```python
from build123d import *

# Parameters (mm, degrees)
SKETCH8_W           = 75
SKETCH8_H           = 10
BOSS_EXTRUDE5_DEPTH = 10
SKETCH9_R           = 5
BOSS_EXTRUDE7_DEPTH = 25
CUT_EXTRUDE1_DEPTH  = 84.366660003
CHAMFER1_SIZE       = 1
FILLET1_R           = 1


with BuildPart() as part:
    # Sketch8 → Boss-Extrude5 (new body)
    with BuildSketch(Plane(origin=(0, 0, 0), x_dir=(1, 0, 0), z_dir=(0, 1, 0))):
        with Locations((-37.5, -5)):
            Rectangle(SKETCH8_W, SKETCH8_H)
    extrude(amount=BOSS_EXTRUDE5_DEPTH)

    # Sketch9 → Boss-Extrude7 (add)
    with BuildSketch(Plane(origin=(0, 10, 0), x_dir=(1, 0, 0), z_dir=(0, 1, 0))):
        with Locations(Location((-70, -5, 0), (0, 0, 270))):
            Circle(SKETCH9_R)
    extrude(amount=BOSS_EXTRUDE7_DEPTH)

    # Sketch13 → Cut-Extrude1 (cut, through all)
    with BuildSketch(Plane.XY.offset(10)):
        with BuildLine():
            Line((-3.73, 6.977270846), (-6.27, 6.977270846))
            ThreePointArc((-6.27, 6.977270846), (-6.126499001, 2.937598487), (-2.65, 5))
            ThreePointArc((-2.65, 5), (-2.937598487, 6.126499001), (-3.73, 6.977270846))
        make_face()
    extrude(amount=-CUT_EXTRUDE1_DEPTH, mode=Mode.SUBTRACT)

    # Chamfer1
    # the kernel refuses this chamfer: 1 mm, written as the material it takes off along each edge
    with BuildSketch(Plane(origin=(-74.333333333, 9.333333333, 0.666666667), x_dir=(-0.7071067811865476, 0, 0.7071067811865475), z_dir=(-0.5773502691896257, 0.5773502691896256, -0.5773502691896258)), Plane(origin=(-74.333333333, 9.333333333, 9.333333333), x_dir=(0, 0.7071067811865475, -0.7071067811865475), z_dir=(-0.5773502691896258, 0.5773502691896258, 0.5773502691896258)), Plane(origin=(-0.666666667, 9.333333333, 9.333333333), x_dir=(0.7071067811865479, 0, -0.7071067811865471), z_dir=(0.5773502691896254, 0.577350269189626, 0.577350269189626)), Plane(origin=(-74.333333333, 0.666666667, 0.666666667), x_dir=(0, -0.7071067811865476, 0.7071067811865476), z_dir=(-0.5773502691896256, -0.5773502691896258, -0.5773502691896258)), Plane(origin=(-0.666666667, 0.666666667, 0.666666667), x_dir=(0.7071067811865476, 0, 0.7071067811865475), z_dir=(0.5773502691896257, -0.5773502691896257, -0.5773502691896258))) as chamfer1_piece_1:
        Polygon((-0.707106781, -0.40824829), (0.707106781, -0.40824829), (0, 0.816496581), align=None)
    extrude(amount=1.270170592, mode=Mode.SUBTRACT)
    with BuildSketch(Plane(origin=(-0.666666667, 9.333333333, 0.666666667), x_dir=(0.7071067811865476, 0, 0.7071067811865475), z_dir=(0.5773502691896257, 0.5773502691896257, -0.5773502691896258)), Plane(origin=(-74.333333333, 0.666666667, 9.333333333), x_dir=(0, -0.7071067811865475, -0.7071067811865476), z_dir=(-0.5773502691896256, -0.5773502691896258, 0.5773502691896257)), Plane(origin=(-0.666666667, 0.666666667, 9.333333333), x_dir=(0.7071067811865479, 0, -0.7071067811865471), z_dir=(0.5773502691896253, -0.577350269189626, 0.5773502691896258))) as chamfer1_piece_2:
        Polygon((-0.707106781, 0.40824829), (0.707106781, 0.40824829), (0, -0.816496581), align=None)
    extrude(amount=1.270170592, mode=Mode.SUBTRACT)
    with BuildSketch(Plane(origin=(-75, 10, -2.571682988), x_dir=(-0.0274958766105822, -0.999621916911297, 0), z_dir=(0, 0, 1))) as chamfer1_piece_3_section:
        Polygon((CHAMFER1_SIZE * 0.999621916911, CHAMFER1_SIZE * 0.0274958766106), (-CHAMFER1_SIZE * 0.0274958766106, CHAMFER1_SIZE * 0.999621916911), (0, 0), align=None)
    chamfer1_piece_3 = extrude(amount=7.571682988, mode=Mode.PRIVATE)
    chamfer1_piece_3 = chamfer1_piece_3 - Plane(origin=(-70, 9.64391603, 5), x_dir=(0, 0, 1), z_dir=(0, -1, 0)) * Cylinder(5, 20, mode=Mode.PRIVATE)
    add(chamfer1_piece_3, mode=Mode.SUBTRACT)
    with BuildSketch(Plane(origin=(-77.571682988, 10, 10), x_dir=(0, -0.9996219169112968, 0.027495876610585647), z_dir=(1, 0, 0))) as chamfer1_piece_4_section:
        Polygon((CHAMFER1_SIZE * 0.999621916911, CHAMFER1_SIZE * 0.0274958766106), (-CHAMFER1_SIZE * 0.0274958766106, CHAMFER1_SIZE * 0.999621916911), (0, 0), align=None)
    chamfer1_piece_4 = extrude(amount=7.571682988, mode=Mode.PRIVATE)
    chamfer1_piece_4 = chamfer1_piece_4 - Plane(origin=(-70, 9.64391603, 5), x_dir=(0, 0, 1), z_dir=(0, -1, 0)) * Cylinder(5, 20, mode=Mode.PRIVATE)
    add(chamfer1_piece_4, mode=Mode.SUBTRACT)
    with BuildSketch(Plane(origin=(-69.999999992, 10, 0), x_dir=(0, -0.9996219169112968, -0.0274958766105864), z_dir=(-1, 0, 0))) as chamfer1_piece_5_section:
        Polygon((CHAMFER1_SIZE * 0.999621916911, CHAMFER1_SIZE * 0.0274958766106), (-CHAMFER1_SIZE * 0.0274958766106, CHAMFER1_SIZE * 0.999621916911), (0, 0), align=None)
    chamfer1_piece_5 = extrude(amount=7.571682996, mode=Mode.PRIVATE)
    chamfer1_piece_5 = chamfer1_piece_5 - Plane(origin=(-70, 9.643916029, 5), x_dir=(0, 0, 1), z_dir=(0, -1, 0)) * Cylinder(5, 20, mode=Mode.PRIVATE)
    add(chamfer1_piece_5, mode=Mode.SUBTRACT)
    with BuildSketch(Plane(origin=(-75, 10, 5), x_dir=(-0.0274958766105822, -0.999621916911297, 0), z_dir=(0, 0, 1))) as chamfer1_piece_6_section:
        Polygon((CHAMFER1_SIZE * 0.999621916911, CHAMFER1_SIZE * 0.0274958766106), (-CHAMFER1_SIZE * 0.0274958766106, CHAMFER1_SIZE * 0.999621916911), (0, 0), align=None)
    chamfer1_piece_6 = extrude(amount=7.571682988, mode=Mode.PRIVATE)
    chamfer1_piece_6 = chamfer1_piece_6 - Plane(origin=(-70, 9.643916029, 5), x_dir=(0, 0, 1), z_dir=(0, -1, 0)) * Cylinder(5, 20, mode=Mode.PRIVATE)
    add(chamfer1_piece_6, mode=Mode.SUBTRACT)
    with BuildSketch(Plane(origin=(-70, 10, 10), x_dir=(0, 0.027495876610585647, -0.9996219169112968), z_dir=(1, 0, 0))) as chamfer1_piece_7_section:
        Polygon((CHAMFER1_SIZE * 0.999621916911, -CHAMFER1_SIZE * 0.0274958766106), (-CHAMFER1_SIZE * 0.0274958766106, -CHAMFER1_SIZE * 0.999621916911), (0, 0), align=None)
    chamfer1_piece_7 = extrude(amount=72.571682988, mode=Mode.PRIVATE)
    chamfer1_piece_7 = chamfer1_piece_7 - Plane(origin=(-70, 9.665551568, 5), x_dir=(0, 0, 1), z_dir=(0, -1, 0)) * Cylinder(5, 150, mode=Mode.PRIVATE)
    add(chamfer1_piece_7, mode=Mode.SUBTRACT)
    with BuildSketch(Plane(origin=(0, 10, 12.571682988), x_dir=(0.027495876610586414, -0.9996219169112968, 0), z_dir=(0, 0, -1)), Plane(origin=(-75, 0, -2.571682988), x_dir=(0.9996219169112968, -0.027495876610586483, 0), z_dir=(0, 0, 1)), Plane(origin=(0, -2.571682988, 10), x_dir=(0.02749587661058629, 0, -0.9996219169112968), z_dir=(0, 1, 0)), Plane(origin=(0, -2.571682988, 0), x_dir=(-0.9996219169112968, 0, -0.02749587661058625), z_dir=(0, 1, 0))) as chamfer1_piece_8:
        Polygon((CHAMFER1_SIZE * 0.999621916911, CHAMFER1_SIZE * 0.0274958766106), (-CHAMFER1_SIZE * 0.0274958766106, CHAMFER1_SIZE * 0.999621916911), (0, 0), align=None)
    extrude(amount=15.143365976, mode=Mode.SUBTRACT)
    with BuildSketch(Plane(origin=(-77.571682988, 0, 10), x_dir=(0, -0.02749587661058639, -0.9996219169112968), z_dir=(1, 0, 0))) as chamfer1_piece_9:
        Polygon((CHAMFER1_SIZE * 0.999621916911, CHAMFER1_SIZE * 0.0274958766106), (-CHAMFER1_SIZE * 0.0274958766106, CHAMFER1_SIZE * 0.999621916911), (0, 0), align=None)
    extrude(amount=80.143365976, mode=Mode.SUBTRACT)
    with BuildSketch(Plane(origin=(2.571682988, 0, 0), x_dir=(0, 0.9996219169112968, -0.027495876610586382), z_dir=(-1, 0, 0))) as chamfer1_piece_10:
        Polygon((CHAMFER1_SIZE * 0.999621916911, -CHAMFER1_SIZE * 0.0274958766106), (-CHAMFER1_SIZE * 0.0274958766106, -CHAMFER1_SIZE * 0.999621916911), (0, 0), align=None)
    extrude(amount=80.143365976, mode=Mode.SUBTRACT)
    with BuildSketch(Plane(origin=(0, 0, 12.571682988), x_dir=(0.027495876610586393, 0.9996219169112968, 0), z_dir=(0, 0, -1)), Plane(origin=(-75, -2.571682988, 10), x_dir=(-0.0274958766105822, 0, -0.999621916911297), z_dir=(0, 1, 0)), Plane(origin=(-75, -2.571682988, 0), x_dir=(0.9996219169112968, 0, -0.0274958766105866), z_dir=(0, 1, 0))) as chamfer1_piece_11:
        Polygon((CHAMFER1_SIZE * 0.999621916911, -CHAMFER1_SIZE * 0.0274958766106), (-CHAMFER1_SIZE * 0.0274958766106, -CHAMFER1_SIZE * 0.999621916911), (0, 0), align=None)
    extrude(amount=15.143365976, mode=Mode.SUBTRACT)
    with BuildSketch(Plane(origin=(2.571682988, 10, 0), x_dir=(0, -0.9996219169112968, -0.0274958766105864), z_dir=(-1, 0, 0))) as chamfer1_piece_12_section:
        Polygon((CHAMFER1_SIZE * 0.999621916911, CHAMFER1_SIZE * 0.0274958766106), (-CHAMFER1_SIZE * 0.0274958766106, CHAMFER1_SIZE * 0.999621916911), (0, 0), align=None)
    chamfer1_piece_12 = extrude(amount=72.571682979, mode=Mode.PRIVATE)
    chamfer1_piece_12 = chamfer1_piece_12 - Plane(origin=(-70, 9.665551567, 5), x_dir=(0, 0, 1), z_dir=(0, -1, 0)) * Cylinder(5, 150, mode=Mode.PRIVATE)
    add(chamfer1_piece_12, mode=Mode.SUBTRACT)

    # Fillet1
    fillet1_edges = [part.edges().sort_by_distance(p)[0] for p in [
        (-70, 35, 0),
    ]]
    fillet(fillet1_edges, radius=FILLET1_R)


solid = part.part
```
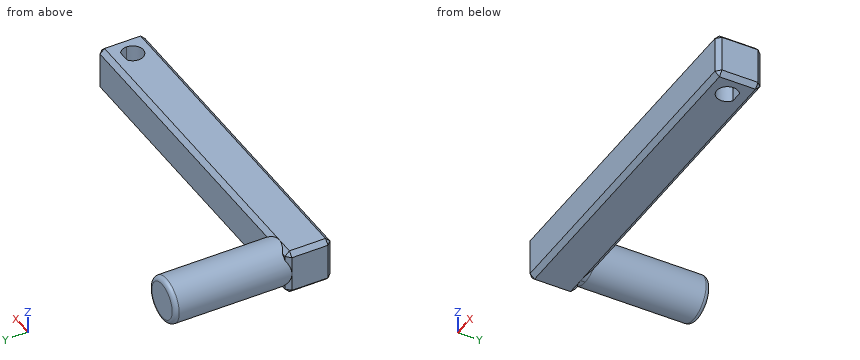
Check sheet for the modelled part. Datum: model origin and axes. Units: mm. Round coordinates to 2 decimals unless told otherwise and drop trailing zeros. Order: outer loops, then holes, each group sorted by start corner. A loop starts at its lowest first (then second) coordinate and runs counter-clockwise, first axis right, second up. Notation, with made-up numbers: M -15.5,-12.5 L 11.5,-12.5 A12 ccw 11.5,5.5 Z; hole C 57.5,6 d5. An arc over 180 degrees is marked long. Answer in a Markdown table with one row per item.
(1) Gauge pin test, flat ends, axial feed: pin 1 (4 mm diameter, centred on x = -19, z = 8, fed in from +Y); pin 2 (12 mm diameter, centred on x = -32, y = 17.5, fed in from -Z); pin 3 (1.1 mm diameter, centred on x = -73.5, z = 8.5, fed in from +Y); pin 4 (0.8 mm diameter, centred on x = -73.5, z = 1.5, fed in from +Y). Record the tip position at first contact, or that the pin passes through.
Findings:
| item | result |
|---|---|
| pin 1 | stops at y = 10 |
| pin 2 | passes through |
| pin 3 | stops at y = 34.92 |
| pin 4 | stops at y = 34.84 |
(2) Material ranges on line 1 along X through (y, z) = (5, 8); line 2 along Y through (x, z) = (-5, 8.25); line 3 along Y through (x, z) = (-8, 8), recorded low to high. Write a range as from..to.
Findings:
| item | result |
|---|---|
| line 1 | x = -75..-7.35, -2.65..0 |
| line 2 | y = 0..2.65, 6.98..10 |
| line 3 | y = 0..10 |
(3) Section check C-C on y = 19.5. Record the boundary of the cut face in (x, z).
Findings:
| item | result |
|---|---|
| outline | C -70,5 d10 |
(4) Section check B-B on x = -36. Record the boundary of the cut face in (y, z).
Findings:
| item | result |
|---|---|
| outline | M 0,1 L 1,0 L 9,0 L 10,1 L 10,9 L 9,10 L 1,10 L 0,9 Z |
(5) Section check A-A on x = -5. Record the boundary of the cut face in (y, z), plus the area to 3 significant figures.
Findings:
| item | result |
|---|---|
| outline | M 0,1 L 1,0 L 2.65,0 L 2.65,10 L 1,10 L 0,9 Z; M 6.98,0 L 9,0 L 10,1 L 10,9 L 9,10 L 6.98,10 Z |
| area | 54.7 mm^2 |
